Design review of the part built by this model. Coordinates are the model's own, in mm. A direction names the side the tool comes from. Coordinates: 2 decimals unless noted, no trailing zeros. Order: outer loops, then holes, each group sorted by start corner. A loop starts at its lowest first (then second) coordinate and runs counter-clockwise, first axis right, second up. Notation, with made-up numbers: (5, 76.25) -> (21, 76.25) arc R29 ccw to (21, 102.25) -> close; hole circle Ø7 at (12, 59.5). An arc over 180 degrees is marked (long way). Write item = value, one per line.
```python
from build123d import *

# Parameters (mm, degrees)
CROQUIS1_W              = 985
CROQUIS1_H              = 150
SALIENTE_EXTRUIR1_DEPTH = 12
CROQUIS2_W              = 600
CROQUIS2_H              = 36
CORTAR_EXTRUIR1_DEPTH   = 9
CROQUIS3_W              = 128.261008082
CROQUIS3_H              = 26
CORTAR_EXTRUIR2_DEPTH   = 13


with BuildPart() as part:
    # Croquis1 → Saliente-Extruir1 (new body)
    with BuildSketch(Plane.XY):
        with Locations((492.5, 75)):
            Rectangle(CROQUIS1_W, CROQUIS1_H)
    extrude(amount=SALIENTE_EXTRUIR1_DEPTH)

    # Croquis2 → Cortar-Extruir1 (cut)
    with BuildSketch(Plane.XY.offset(12)):
        with Locations((336, 114.5)):
            Rectangle(CROQUIS2_W, CROQUIS2_H)
        with Locations((336, 35.5)):
            Rectangle(CROQUIS2_W, CROQUIS2_H)
    extrude(amount=-CORTAR_EXTRUIR1_DEPTH, mode=Mode.SUBTRACT)

    # Croquis3 → Cortar-Extruir2 (cut, through all)
    with BuildSketch(Plane.XY.offset(12)):
        with Locations((74.130504041, 75)):
            Rectangle(CROQUIS3_W, CROQUIS3_H)
    extrude(amount=-CORTAR_EXTRUIR2_DEPTH, mode=Mode.SUBTRACT)


solid = part.part
```
(1) We need section B-B (x = 576). Write out the cut boundary in (y, z), and give its area (3 significant figures).
Report:
outline = (0, 0) -> (150, 0) -> (150, 12) -> (132.5, 12) -> (132.5, 3) -> (96.5, 3) -> (96.5, 12) -> (53.5, 12) -> (53.5, 3) -> (17.5, 3) -> (17.5, 12) -> (0, 12) -> close
area = 1,150 mm²
(2) Insertion check: pin 1 (11 mm diameter, centred on x = 370.5, y = 116, fed in from +Z). The pin has a flat end and moves straight along its axis. Give the tip position at first contact, or say it passes through.
Report:
pin_1 = 3
(3) For faces 3 (the flat face through (332, 36, 3)), 4 (the flat face through (595, 76, 12)), list the 3-axis set-ups (+Z, -Z, +X, -X, +Y, -Y) from which the entire face can be reached by the end or side of a thin tool; tool diameter is ignored.
Report:
face_3 = +Z
face_4 = +Z, +X, -X, +Y, -Y
(4) We need section C-C (y = 40.5). Write out the cut boundary in (x, z), and give its area (3 significant figures).
Report:
outline = (0, 0) -> (985, 0) -> (985, 12) -> (636, 12) -> (636, 3) -> (36, 3) -> (36, 12) -> (0, 12) -> close
area = 6,420 mm²
(5) The part is to be moulded in two halves that separate along X. For faces 1 (the flat face through (332, 115, 3)), 2 (the flat face through (486, 76, 0)), say which applies: released by +X, released by -X, zero draft, split by the parting line, or undercut.
Report:
face_1 = undercut
face_2 = zero draft
(6) We need section A-A (z = 7.5). Write out the cut boundary in (x, y).
Report:
outline = (0, 0) -> (985, 0) -> (985, 150) -> (0, 150) -> close; hole (10, 62) -> (138.26, 62) -> (138.26, 88) -> (10, 88) -> close; hole (36, 17.5) -> (636, 17.5) -> (636, 53.5) -> (36, 53.5) -> close; hole (36, 96.5) -> (636, 96.5) -> (636, 132.5) -> (36, 132.5) -> close
(7) For L1, parallel to Y at x = 522.5, z = 9.25; L2, parallel to Y at x = 109, z = 8.75; L3, parallel to X at y = 77.5, z = 8, list the stretches that pass through material, from the lowest coordinate up.
Report:
L1 = 0 to 17.5, 53.5 to 96.5, 132.5 to 150
L2 = 0 to 17.5, 53.5 to 62, 88 to 96.5, 132.5 to 150
L3 = 0 to 10, 138.26 to 985
